Check sheet for the drawn part. Datum: minimum x, y, z corner. Units: mm. Give positions to 0.01 mm unless a question says otherwise; leave off trailing zeros. Loops run counter-clockwise (first coordinate to the right, second up) from the corner with the lowest first, then second, coordinate; pieces in that order, holes last. Notation, with made-up numbers: (-39.5, 24.25) - (-15.5, 24.25) arc R27 ccw to (-15.5, 61.25) - close; hole circle Ø1 at (3, 49). An arc over 180 degrees is marked (long way). Use one line per item in the form item = value.
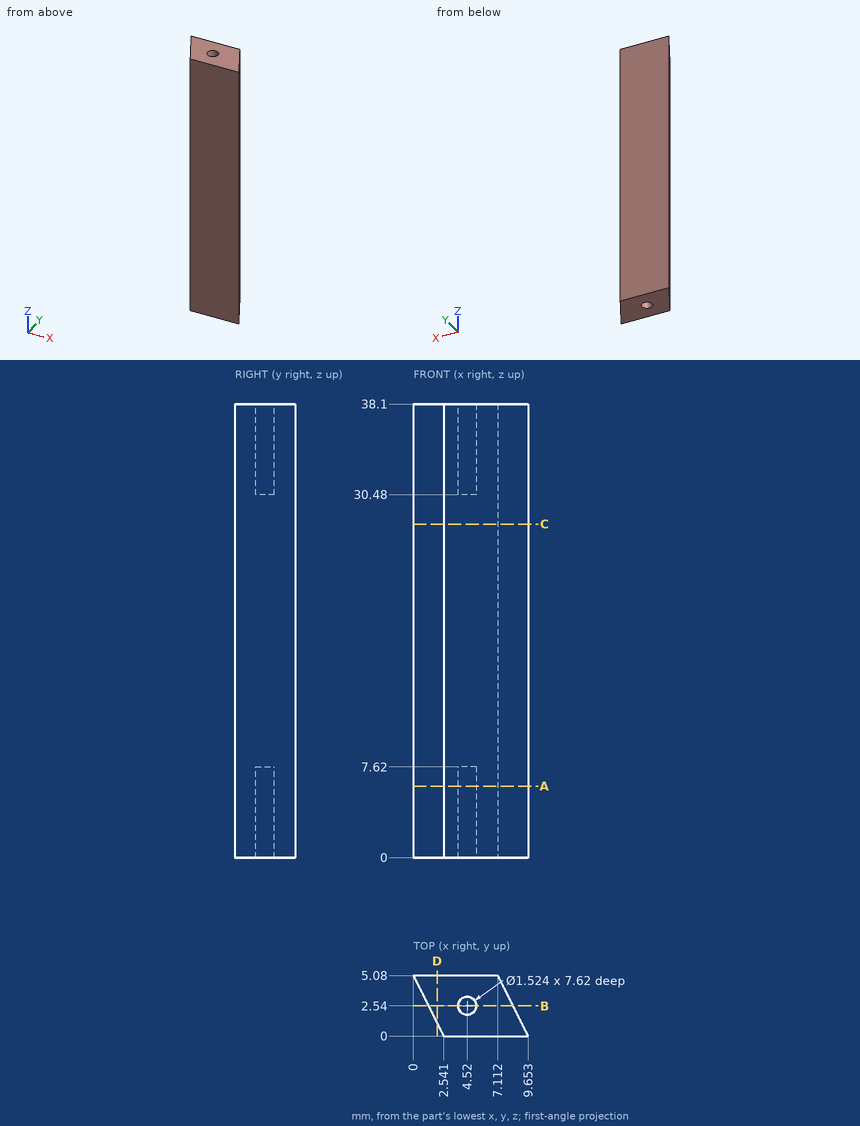
1. Section check C-C, the plane z = 28. Record the cut outline in (x, y).
Result set:
outline = (0, 5.08) - (2.54, 0) - (9.65, 0) - (7.11, 5.08) - close
2. Depth check by flat-ended pin: pin 1 Ø0.5 at (x, y) = (4.5, 3) entering from -Z; pin 2 Ø1.5 at (y, z) = (4, 30) entering from +X; pin 3 Ø0.5 at (x, y) = (4.5, 2.5) entering from +Z. Enter the tip coordinate at first touch or a pass-through.
Result set:
pin_1 = 7.62
pin_2 = 8.03
pin_3 = 30.48
3. Section check D-D, the plane x = 2. Record the cut outline in (y, z), then the cut area to 3 significant figures.
Result set:
outline = (1.08, 0) - (5.08, 0) - (5.08, 38.1) - (1.08, 38.1) - close
area = 152 mm²
4. Section check A-A, the plane z = 6. Record the cut outline in (x, y).
Result set:
outline = (0, 5.08) - (2.54, 0) - (9.65, 0) - (7.11, 5.08) - close; hole circle Ø1.52 at (4.52, 2.54)
5. Scan lines: probe 1 along X at (y, z) = (2.54, 2.75); probe 2 along X at (y, z) = (2.35, 6.5) (1 decimal); probe 3 along Y at (x, z) = (4.75, 4.5) (1 decimal). Record each from-to range of solid material in increasing order.
Result set:
probe_1 = 1.27 to 3.76, 5.28 to 8.38
probe_2 = 1.4 to 3.8, 5.3 to 8.5
probe_3 = 0 to 1.8, 3.3 to 5.1
6. Section check B-B, the plane y = 2.54. Record the cut outline in (x, z), then the cut area to 3 significant figures.
Result set:
outline = (1.27, 0) - (3.76, 0) - (3.76, 7.62) - (5.28, 7.62) - (5.28, 0) - (8.38, 0) - (8.38, 38.1) - (5.28, 38.1) - (5.28, 30.48) - (3.76, 30.48) - (3.76, 38.1) - (1.27, 38.1) - close
area = 248 mm²
